```python
from build123d import *

# Parameters (mm, degrees)
SKETCH1_R           = 1.55
BOSS_EXTRUDE1_DEPTH = 4.8


with BuildPart() as part:
    # Sketch1 → Boss-Extrude1 (new body)
    with BuildSketch(Plane.XY):
        with BuildLine():
            ThreePointArc((-1.220475879, -2.635924597), (-1.222210326, -2.658421079), (-1.225048855, -2.680805064))
            ThreePointArc((-1.225048855, -2.680805064), (-1.237827813, -2.990086384), (-1.183146697, -3.294763611))
            ThreePointArc((-1.183146697, -3.294763611), (-0.986277373, -3.358952263), (-0.785957353, -3.411388925))
            ThreePointArc((-0.785957353, -3.411388925), (-0.575235727, -3.184640974), (-0.418775964, -2.917548145))
            ThreePointArc((-0.418775964, -2.917548145), (-0.409062191, -2.897182914), (-0.398358784, -2.877319956))
            ThreePointArc((-0.398358784, -2.877319956), (0, -2.646063949), (0.398358784, -2.877319957))
            ThreePointArc((0.398358784, -2.877319957), (0.409062191, -2.897182914), (0.418775964, -2.917548145))
            ThreePointArc((0.418775964, -2.917548145), (0.575235727, -3.184640974), (0.785957353, -3.411388925))
            ThreePointArc((0.785957353, -3.411388925), (0.986277373, -3.358952263), (1.183146697, -3.294763611))
            ThreePointArc((1.183146697, -3.294763611), (1.237827812, -2.990086385), (1.225048855, -2.680805065))
            ThreePointArc((1.225048855, -2.680805065), (1.222210326, -2.65842108), (1.220475879, -2.635924598))
            ThreePointArc((1.220475879, -2.635924598), (1.430570178, -2.226010644), (1.890717351, -2.205186558))
            ThreePointArc((1.890717351, -2.205186558), (1.910460355, -2.216109643), (1.929642376, -2.227990303))
            ThreePointArc((1.929642376, -2.227990303), (2.205665989, -2.368094556), (2.505525497, -2.444922359))
            ThreePointArc((2.505525497, -2.444922359), (2.645696022, -2.292508653), (2.776610031, -2.13207413))
            ThreePointArc((2.776610031, -2.13207413), (2.657889767, -1.846200494), (2.479929318, -1.592925316))
            ThreePointArc((2.479929318, -1.592925316), (2.4654397, -1.575629335), (2.451818074, -1.557641803))
            ThreePointArc((2.451818074, -1.557641803), (2.40694443, -1.09921469), (2.782786513, -0.832922011))
            ThreePointArc((2.782786513, -0.832922011), (2.80530085, -0.831437221), (2.827860963, -0.831061285))
            ThreePointArc((2.827860963, -0.831061285), (3.135812881, -0.79969485), (3.429606999, -0.702210219))
            ThreePointArc((3.429606999, -0.702210219), (3.465124877, -0.498209743), (3.488519299, -0.292466177))
            ThreePointArc((3.488519299, -0.292466177), (3.234090501, -0.116158991), (2.947449745, 0.000696964))
            ThreePointArc((2.947449745, 0.000696964), (2.925909389, 0.00741359), (2.904725354, 0.015181258))
            ThreePointArc((2.904725354, 0.015181258), (2.619130834, 0.376574163), (2.791340622, 0.80378939))
            ThreePointArc((2.791340622, 0.80378939), (2.80947815, 0.817210645), (2.828253678, 0.829723821))
            ThreePointArc((2.828253678, 0.829723821), (3.070361342, 1.022602322), (3.264812511, 1.263448704))
            ThreePointArc((3.264812511, 1.263448704), (3.184401067, 1.454267239), (3.092848337, 1.63999772))
            ThreePointArc((3.092848337, 1.63999772), (2.783490351, 1.65076217), (2.479175704, 1.594097963))
            ThreePointArc((2.479175704, 1.594097963), (2.457423521, 1.588102753), (2.435402858, 1.583184377))
            ThreePointArc((2.435402858, 1.583184377), (1.999761704, 1.73280338), (1.913663807, 2.18530334))
            ThreePointArc((1.913663807, 2.18530334), (1.921665988, 2.206399906), (1.930695833, 2.227077476))
            ThreePointArc((1.930695833, 2.227077476), (2.030091771, 2.520230481), (2.063463119, 2.82797159))
            ThreePointArc((2.063463119, 2.82797159), (1.892652419, 2.945024649), (1.715219882, 3.051773929))
            ThreePointArc((1.715219882, 3.051773929), (1.449151682, 2.893578006), (1.223780893, 2.681384122))
            ThreePointArc((1.223780893, 2.681384122), (1.208723048, 2.664580512), (1.192857163, 2.648537642))
            ThreePointArc((1.192857163, 2.648537642), (0.745482362, 2.538879767), (0.428412254, 2.87299892))
            ThreePointArc((0.428412254, 2.87299892), (0.423738452, 2.895072786), (0.420155704, 2.917349768))
            ThreePointArc((0.420155704, 2.917349768), (0.345282406, 3.217703271), (0.206978766, 3.494633479))
            ThreePointArc((0.206978766, 3.494633479), (0.103534673, 3.499226191), (0, 3.500757541))
            ThreePointArc((0, 3.500757541), (-0.103534673, 3.499226191), (-0.206978766, 3.494633479))
            ThreePointArc((-0.206978766, 3.494633479), (-0.345282406, 3.217703271), (-0.420155704, 2.917349768))
            ThreePointArc((-0.420155704, 2.917349768), (-0.423738452, 2.895072786), (-0.428412254, 2.87299892))
            ThreePointArc((-0.428412254, 2.87299892), (-0.745482362, 2.538879767), (-1.192857163, 2.648537642))
            ThreePointArc((-1.192857163, 2.648537642), (-1.208723048, 2.664580512), (-1.223780893, 2.681384122))
            ThreePointArc((-1.223780893, 2.681384122), (-1.449151682, 2.893578006), (-1.715219882, 3.051773929))
            ThreePointArc((-1.715219882, 3.051773929), (-1.892652419, 2.945024649), (-2.063463119, 2.82797159))
            ThreePointArc((-2.063463119, 2.82797159), (-2.030091771, 2.520230481), (-1.930695833, 2.227077476))
            ThreePointArc((-1.930695833, 2.227077476), (-1.921665988, 2.206399906), (-1.913663807, 2.18530334))
            ThreePointArc((-1.913663807, 2.18530334), (-1.999761704, 1.73280338), (-2.435402858, 1.583184377))
            ThreePointArc((-2.435402858, 1.583184377), (-2.457423521, 1.588102753), (-2.479175704, 1.594097963))
            ThreePointArc((-2.479175704, 1.594097963), (-2.783490351, 1.65076217), (-3.092848337, 1.63999772))
            ThreePointArc((-3.092848337, 1.63999772), (-3.184401067, 1.454267239), (-3.264812511, 1.263448704))
            ThreePointArc((-3.264812511, 1.263448704), (-3.070361342, 1.022602322), (-2.828253678, 0.829723821))
            ThreePointArc((-2.828253678, 0.829723821), (-2.80947815, 0.817210645), (-2.791340622, 0.80378939))
            ThreePointArc((-2.791340622, 0.80378939), (-2.619130834, 0.376574163), (-2.904725354, 0.015181258))
            ThreePointArc((-2.904725354, 0.015181258), (-2.925909389, 0.00741359), (-2.947449745, 0.000696964))
            ThreePointArc((-2.947449745, 0.000696964), (-3.234090501, -0.116158991), (-3.488519299, -0.292466177))
            ThreePointArc((-3.488519299, -0.292466177), (-3.465124877, -0.498209743), (-3.429606999, -0.702210219))
            ThreePointArc((-3.429606999, -0.702210219), (-3.135812881, -0.79969485), (-2.827860963, -0.831061285))
            ThreePointArc((-2.827860963, -0.831061285), (-2.80530085, -0.831437221), (-2.782786513, -0.832922011))
            ThreePointArc((-2.782786513, -0.832922011), (-2.40694443, -1.09921469), (-2.451818074, -1.557641803))
            ThreePointArc((-2.451818074, -1.557641803), (-2.4654397, -1.575629335), (-2.479929318, -1.592925316))
            ThreePointArc((-2.479929318, -1.592925316), (-2.657889767, -1.846200494), (-2.776610031, -2.13207413))
            ThreePointArc((-2.776610031, -2.13207413), (-2.645696022, -2.292508653), (-2.505525497, -2.444922359))
            ThreePointArc((-2.505525497, -2.444922359), (-2.205665987, -2.368094557), (-1.929642373, -2.227990304))
            ThreePointArc((-1.929642373, -2.227990304), (-1.910460352, -2.216109645), (-1.890717348, -2.20518656))
            ThreePointArc((-1.890717348, -2.20518656), (-1.430570177, -2.226010646), (-1.220475879, -2.635924597))
        make_face()
        Circle(SKETCH1_R, mode=Mode.SUBTRACT)
    extrude(amount=BOSS_EXTRUDE1_DEPTH)


solid = part.part
```
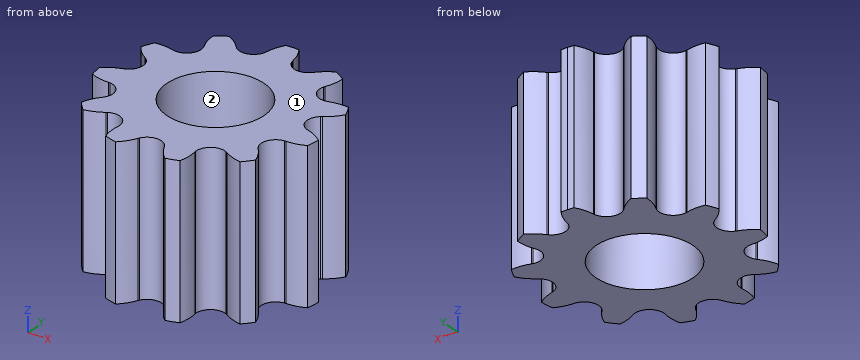
The listing builds one solid part. Answer for the finished solid, in the listing's coordinates (mm). Face numbers are marked on the shaded views. Give positions to 0.01 mm unless a question says otherwise; leave off trailing zeros. Order: outer loops, then holes, each group sorted by start corner. A loop starts at its lowest first (then second) coordinate and runs counter-clockwise, first axis right, second up. Notation, with made-up numbers: (80, 86.5) - (95, 86.5) arc R18 ccw to (95, 120.5) - close; hole circle Ø10 at (60, -31). An arc over 180 degrees is marked (long way). Answer in a Markdown table with one row per item. Add a question column.
Q1. For a pull along Y with two mould halves and no side action, classify the marked faces 1 and 2 as released by +Y, released by -Y, zero draft, split by the parting line, or undercut.
Q2. The part is cut by section C-C (y = 1.75). Determine the outline of the cut face in (x, z), then the cut area to 3 significant figures.
Q3. The part is cut by section A-A (y = -1.25). Determine the outline of the cut face in (x, z), then the cut area to 3 significant figures.
Q4. Find the intervals of material crossed by line 1 along Y through (x, z) = (0, 3.4); line 2 along X through (y, z) = (3, 4.4); line 3 along X through (y, z) = (2.75, 3.7), in increasing order. Write a range as [from, to].
Q5. The part is cut by section D-D (y = 3.25). Determine the outline of the cut face in (x, z), then the cut area to 3 significant figures.
Q6. The part is cut by section B-B (x = -1). Determine the outline of the cut face in (y, z).
Q7. Given P1, Ø1.9, axis at x = 0, y = 0, coming from the -Z side; P2, Ø3, axis at x = 1, y = -1, coming from the +Z side; P3, Ø1, axis at x = 1, z = 1, coming from the +Y side; P4, Ø1.5, axis at x = 2, z = 1, coming from the +Y side, each flat-ended and moving along its own axis, determine where each tip first touches the part or whether it passes through.
Determined:
| question | item | result |
|---|---|---|
| 1 | face 1 | zero draft |
| 1 | face 2 | undercut |
| 2 | outline | (-1.99, 0) - (1.99, 0) - (1.99, 4.8) - (-1.99, 4.8) - close |
| 2 | area | 19.1 mm² |
| 3 | outline | (-2.37, 0) - (-0.92, 0) - (-0.92, 4.8) - (-2.37, 4.8) - close; (0.92, 0) - (2.37, 0) - (2.37, 4.8) - (0.92, 4.8) - close |
| 3 | area | 13.9 mm² |
| 4 | line 1 | y = [-2.65, -1.55], [1.55, 3.5] |
| 4 | line 2 | x = [-1.8, -1.61], [-0.41, 0.41], [1.61, 1.8] |
| 4 | line 3 | x = [-2.06, -1.29], [-0.48, 0.48], [1.29, 2.06] |
| 5 | outline | (-0.33, 0) - (0.33, 0) - (0.33, 4.8) - (-0.33, 4.8) - close |
| 5 | area | 3.20 mm² |
| 6 | outline | (-3.35, 0) - (-1.18, 0) - (-1.18, 4.8) - (-3.35, 4.8) - close; (1.18, 0) - (2.54, 0) - (2.54, 4.8) - (1.18, 4.8) - close |
| 7 | P1 | passes through |
| 7 | P2 | stops at z = 4.8 |
| 7 | P3 | stops at y = 2.93 |
| 7 | P4 | stops at y = 3.05 |
